```python
from build123d import *

# Parameters (mm, degrees)
BOSS_EXTRUDE1_DEPTH     = 2
SKETCH2_W               = 110.931662833
SKETCH2_H               = 3
SKETCH2_W_2             = 124.512387616
SKETCH2_W_3             = 131.50444394
SKETCH2_W_4             = 133.924771129
CUT_EXTRUDE1_DEPTH      = 0.5
CUT_EXTRUDE3_DEPTH      = 102.262036322
CUT_EXTRUDE3_DEPTH_BACK = 102.262036322
SKETCH3_W               = 29
SKETCH3_H               = 20
FILLET1_R               = 1


with BuildPart() as part:
    # Sketch1 → Boss-Extrude1 (new body)
    with BuildSketch(Plane(origin=(0, 0, 0), x_dir=(1, 0, 0), z_dir=(0, 1, 0))):
        with BuildLine():
            Line((0, 35), (-60, 35))
            ThreePointArc((-60, 35), (-95, 0), (-60, -35))
            Line((-60, -35), (0, -35))
            ThreePointArc((0, -35), (35, 0), (0, 35))
        make_face()
    extrude(amount=BOSS_EXTRUDE1_DEPTH)

    # Sketch2 → Cut-Extrude1 (cut)
    with BuildSketch(Plane(origin=(0, 2, 0), x_dir=(1, 0, 0), z_dir=(0, 1, 0))):
        with Locations((-30.336156555, 28.5)):
            Rectangle(SKETCH2_W, SKETCH2_H)
        with Locations((-30, 20.5)):
            Rectangle(SKETCH2_W_2, SKETCH2_H)
        with Locations((-29.865537378, 12.5)):
            Rectangle(SKETCH2_W_3, SKETCH2_H)
        with Locations((-28.655373784, 4.5)):
            Rectangle(SKETCH2_W_4, SKETCH2_H)
        with Locations((-28.655373784, -4.5)):
            Rectangle(SKETCH2_W_4, SKETCH2_H)
        with Locations((-29.865537378, -12.5)):
            Rectangle(SKETCH2_W_3, SKETCH2_H)
        with Locations((-30, -20.5)):
            Rectangle(SKETCH2_W_2, SKETCH2_H)
        with Locations((-30.336156555, -28.5)):
            Rectangle(SKETCH2_W, SKETCH2_H)
    extrude(amount=-CUT_EXTRUDE1_DEPTH, mode=Mode.SUBTRACT)

    # Sketch3 → Cut-Extrude3 (cut, two sides: drawn at the far end of the back side and taken through both)
    with BuildSketch(Plane(origin=(0, 0, 0), x_dir=(1, 0, 0), z_dir=(0, 1, 0)).offset(-CUT_EXTRUDE3_DEPTH_BACK)):
        with Locations((-74.5, -16.892498432)):
            Rectangle(SKETCH3_W, SKETCH3_H)
    extrude(amount=CUT_EXTRUDE3_DEPTH + CUT_EXTRUDE3_DEPTH_BACK, mode=Mode.SUBTRACT)

    # Fillet1
    fillet1_edges = [part.edges().sort_by_distance(p)[0] for p in [
        (-60, 1, 6.892498432),
        (-89, 1, 6.892498432),
        (-60, 1, 26.892498432),
    ]]
    fillet(fillet1_edges, radius=FILLET1_R)


solid = part.part
```
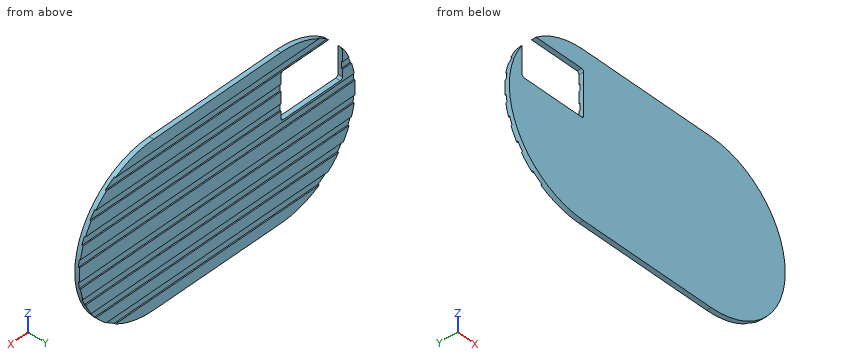
Build history of the part. All positions in model axes, mm. Coordinates: 2 decimals unless noted, no trailing zeros. Write each loop counter-clockwise with the first axis right and the second up, starting at its lowest first coordinate (ties: lowest second). Pieces come first, ordered by that corner, then holes.
1. Drill centre lines: probe 1 along Z at (x, y) = (-78, 0.9); probe 2 along Z at (x, y) = (18, 0.1); probe 3 along Y at (x, z) = (-4.5, -12). Where is each one in solid material? Low to high.
Answer block:
probe 1: z = -30.02 to 6.89, 26.89 to 30.02
probe 2: z = -30.02 to 30.02
probe 3: y = 0 to 1.5
2. Drop flat-ended pins along their axis: pin 1 (3.5 mm diameter, centred on x = 2.5, z = 13, fed in from +Y); pin 2 (1.5 mm diameter, centred on x = -92, z = 12.5, fed in from +Y); pin 3 (0.6 mm diameter, centred on x = -90.5, y = 1.5, fed in from -Z); pin 4 (1 mm diameter, centred on y = 1.5, z = 11.5, fed in from +X). Give the stop position or say it passes through.
Answer block:
pin 1: stops at y = 2
pin 2: stops at y = 1.5
pin 3: stops at z = -17.69
pin 4: stops at x = 33.23
3. Band-saw the part on C-C, the plane z = 23.5. Give the cut face in (x, y), and give its area (3 significant figures).
Answer block:
outline: (-60, 0) - (25.94, 0) - (25.94, 2) - (-60, 2) - close
area: 172 mm2
4. Band-saw the part on A-A, the plane y = 0.5. Give the cut face in (x, z).
Answer block:
outline: (-89, 7.89) - (-89, 19.6) arc R35 ccw to (-60, -35) - (0, -35) arc R35 ccw to (0, 35) - (-60, 35) arc R35 ccw to (-82.4, 26.89) - (-61, 26.89) arc R1 cw to (-60, 25.89) - (-60, 7.89) arc R1 cw to (-61, 6.89) - (-88, 6.89) arc R1 cw to start
